```python
from build123d import *

# Parameters (mm, degrees)
SKETCH1_R           = 67.15
BOSS_EXTRUDE1_DEPTH = 10
SKETCH1_3_R         = 30.48
BOSS_EXTRUDE2_DEPTH = 2
FILLET1_R           = 8
SKETCH2_R           = 2.775
CUT_EXTRUDE1_DEPTH  = 3
CUT_EXTRUDE2_REACH  = 97.39
SKETCH3_R           = 1.6


with BuildPart() as part:
    # Sketch1 → Boss-Extrude1 (new body)
    with BuildSketch(Plane(origin=(0, 0, 0), x_dir=(1, 0, 0), z_dir=(0, 1, 0))):
        with Locations(Location((0, 0, 0), (0, 0, 270))):
            Circle(SKETCH1_R)
    extrude(amount=BOSS_EXTRUDE1_DEPTH)

    # Sketch1_3 → Boss-Extrude2 (add)
    with BuildSketch(Plane(origin=(0, 0, 0), x_dir=(1, 0, 0), z_dir=(0, 1, 0))):
        with Locations(Location((0, 0, 0), (0, 0, 270))):
            Circle(SKETCH1_3_R)
    extrude(amount=-BOSS_EXTRUDE2_DEPTH)

    # Fillet1
    fillet1_edges = [part.edges().sort_by_distance(p)[0] for p in [
        (0, 10, -67.15),
    ]]
    fillet(fillet1_edges, radius=FILLET1_R)

    # Sketch2 → Cut-Extrude1 (cut)
    with BuildSketch(Plane(origin=(0, 10, 0), x_dir=(1, 0, 0), z_dir=(0, 1, 0))):
        with Locations(Location((0, 0, 0), (0, 0, 270))):
            Circle(SKETCH2_R)
    extrude(amount=-CUT_EXTRUDE1_DEPTH, mode=Mode.SUBTRACT)

    # Sketch3 → Cut-Extrude2 (cut, up to next)
    with BuildSketch(Plane(origin=(0, 7, 0), x_dir=(1, 0, 0), z_dir=(0, 1, 0)), mode=Mode.PRIVATE) as cut_extrude2_sk1:
        with Locations(Location((0, 0, 0), (0, 0, 270))):
            Circle(SKETCH3_R)
    cut_extrude2_tool1 = extrude(cut_extrude2_sk1.sketch, amount=-CUT_EXTRUDE2_REACH, mode=Mode.PRIVATE) & part.part
    add(cut_extrude2_tool1.solids().sort_by_distance((0, 7, 0))[0], mode=Mode.SUBTRACT)


solid = part.part
```
Build history of the part. All positions in model axes, mm. A direction names the side the tool comes from. Round coordinates to 2 decimals unless told otherwise and drop trailing zeros. Order: outer loops, then holes, each group sorted by start corner. A loop starts at its lowest first (then second) coordinate and runs counter-clockwise, first axis right, second up. Notation, with made-up numbers: (79, -20.5) - (120, -20.5) arc R21 ccw to (120, 2.5) - close; hole circle Ø1 at (-25.5, 2). An arc over 180 degrees is marked (long way). Use a Markdown table: item, result.
1) Saw through at A-A on x = 0. Write the cut outline in (y, z) (3 decimals), and give its area (3 significant figures).
Recorded:
| item | result |
|---|---|
| outline | (-2, -30.48) - (0, -30.48) - (0, -67.15) - (2, -67.15) arc R8 ccw to (10, -59.15) - (10, -2.775) - (7, -2.775) - (7, -1.6) - (-2, -1.6) - close; (-2, 1.6) - (7, 1.6) - (7, 2.775) - (10, 2.775) - (10, 59.15) arc R8 ccw to (2, 67.15) - (0, 67.15) - (0, 30.48) - (-2, 30.48) - close |
| area | 1,390 mm² |
2) Flat gauge pins, fed straight in: pin 1 Ø3 at (y, z) = (8.5, 52.5) entering from -X; pin 2 Ø1 at (x, y) = (12, 4) entering from -Z; pin 3 Ø1 at (x, z) = (10.5, 49.5) entering from -Y. Where does each tip first touch, or does it go through?
Recorded:
| item | result |
|---|---|
| pin 1 | stops at x = -39.77 |
| pin 2 | stops at z = -65.96 |
| pin 3 | stops at y = 0 |
3) Tool access for faces 4 (the face through (2.34, 8.52, 1.49)), 5 (the face through (-12, 10, -1)), 6 (the face through (30.22, -0.99, -3.97)): list every direction of +Z, -Z, +X, -X, +Y, -Y with a clear straight run to the whole face (end or side of a thin tool).
Recorded:
| item | result |
|---|---|
| face 4 | +Y |
| face 5 | +Z, -Z, +X, -X, +Y |
| face 6 | -Y |
4) Saw through at B-B on z = 0. Write the cut outline in (x, y) (3 decimals).
Recorded:
| item | result |
|---|---|
| outline | (-67.15, 0) - (-30.48, 0) - (-30.48, -2) - (-1.6, -2) - (-1.6, 7) - (-2.775, 7) - (-2.775, 10) - (-59.15, 10) arc R8 ccw to (-67.15, 2) - close; (1.6, -2) - (30.48, -2) - (30.48, 0) - (67.15, 0) - (67.15, 2) arc R8 ccw to (59.15, 10) - (2.775, 10) - (2.775, 7) - (1.6, 7) - close |
5) Saw through at C-C on y = 4. Write the cut outline in (x, z).
Recorded:
| item | result |
|---|---|
| outline | circle Ø133.79 at (0, 0); hole circle Ø3.2 at (0, 0) |
6) Pull direction Z, two halves, no side cores. Call faces 1 (the face through (-0.97, 2.56, -1.27)), 2 (the face through (-6, -2, 0)), 3 (the face through (20.17, 0.99, 64.05)): pulls with the +Z half, pulls with the -Z half, needs draft (parallel to the pull), parting line crosses it, or undercut.
Recorded:
| item | result |
|---|---|
| face 1 | undercut |
| face 2 | needs draft |
| face 3 | parting line crosses it |
7) Wall check: L1, parallel to X at y = 1.5, z = 0; L2, parallel to Y at x = 40, z = 37; L3, parallel to X at y = 5, z = 0. Give the ranges that are in metal, low to high.
Recorded:
| item | result |
|---|---|
| L1 | x = -67.15 to -1.6, 1.6 to 67.15 |
| L2 | y = 0 to 10 |
| L3 | x = -66.57 to -1.6, 1.6 to 66.57 |
